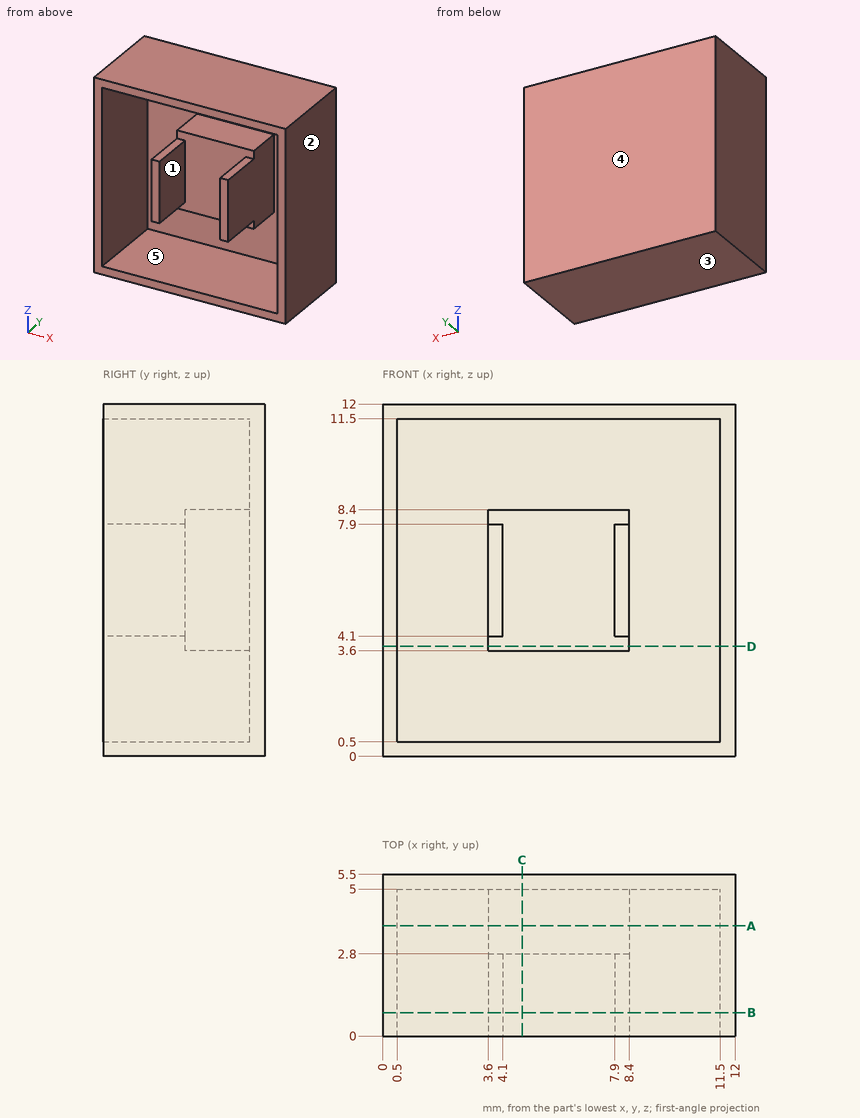
The figure shows three views and two pictorial views of one solid part (mm, origin at its lowest corner). Answer the questions. A direction names the side the tool comes from. Coordinates: 2 decimals unless noted, no trailing zeros. Write each loop counter-clockwise with the first axis right and the second up, starting at its lowest first coordinate (ties: lowest second). Pieces come first, ordered by that corner, then holes. Notation, with made-up numbers: (11.5, 51.5) -> (33.5, 51.5) arc R31 cw to (33.5, 85.5) -> close; hole circle Ø2 at (25, 77). An arc over 180 degrees is marked (long way). Return JSON: item names as keys, results as strings.
1. A cutting plane is placed at A-A (y = 3.75). Determine the outline of the cut face in (x, z).
Found:
{"outline": "(0, 0) -> (12, 0) -> (12, 12) -> (0, 12) -> close; (3.6, 3.6) -> (8.4, 3.6) -> (8.4, 8.4) -> (3.6, 8.4) -> close; hole (0.5, 0.5) -> (11.5, 0.5) -> (11.5, 11.5) -> (0.5, 11.5) -> close"}
2. A tool of negligible diameter and unlimited length cuts with its end or side. For the marked faces 4 and 5, from which of +Z, -Z, +X, -X, +Y, -Y can it reach the whole face along a straight path? Write none if from no direction.
Found:
{"face 4": "+Z, -Z, +X, -X, +Y", "face 5": "-Y"}
3. Determine the mould class of the marked faces 1, 2 and 3 for opening direction Z: pulls with the +Z half, pulls with the -Z half, needs draft (parallel to the pull), parting line crosses it, or undercut.
Found:
{"face 1": "undercut", "face 2": "needs draft", "face 3": "pulls with the -Z half"}
4. This flat-tipped pin is pushed along its axis until it touches: P1, Ø1, axis at x = 2.5, z = 5.5, coming from the -Y side. Where does it stop, or does it pass through?
Found:
{"P1": "y = 5"}
5. A cutting plane is placed at B-B (y = 0.8). Determine the outline of the cut face in (x, z).
Found:
{"outline": "(0, 0) -> (12, 0) -> (12, 12) -> (0, 12) -> close; (3.6, 4.1) -> (4.1, 4.1) -> (4.1, 7.9) -> (3.6, 7.9) -> close; (7.9, 4.1) -> (8.4, 4.1) -> (8.4, 7.9) -> (7.9, 7.9) -> close; hole (0.5, 0.5) -> (11.5, 0.5) -> (11.5, 11.5) -> (0.5, 11.5) -> close"}
6. A cutting plane is placed at C-C (x = 4.75). Determine the outline of the cut face in (y, z).
Found:
{"outline": "(0, 0) -> (5.5, 0) -> (5.5, 12) -> (0, 12) -> (0, 11.5) -> (5, 11.5) -> (5, 8.4) -> (2.8, 8.4) -> (2.8, 3.6) -> (5, 3.6) -> (5, 0.5) -> (0, 0.5) -> close"}
7. A cutting plane is placed at D-D (z = 3.75). Determine the outline of the cut face in (x, y), and give its area (3 significant figures).
Found:
{"outline": "(0, 0) -> (0.5, 0) -> (0.5, 5) -> (3.6, 5) -> (3.6, 2.8) -> (8.4, 2.8) -> (8.4, 5) -> (11.5, 5) -> (11.5, 0) -> (12, 0) -> (12, 5.5) -> (0, 5.5) -> close", "area": "21.6 mm2"}
8. Find the intervals of material crossed by line 1 along X through (y, z) = (3.6, 4); line 2 along X through (y, z) = (2.3, 6.25), in increasing order. Write a range as from..to.
Found:
{"line 1": "0..0.5, 3.6..8.4, 11.5..12", "line 2": "0..0.5, 3.6..4.1, 7.9..8.4, 11.5..12"}
